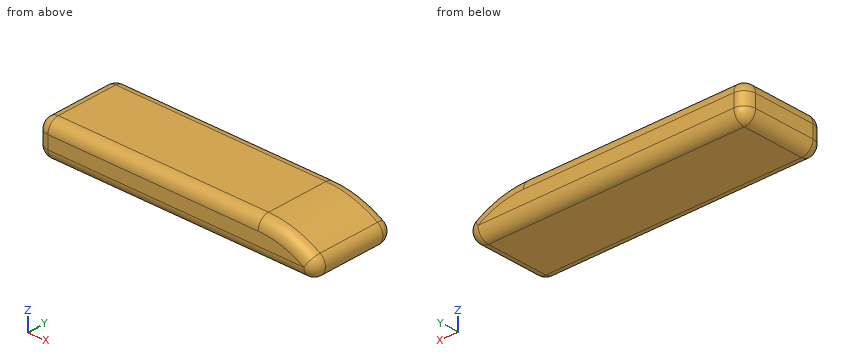
```python
from build123d import *

# Parameters (mm, degrees)
F1_DEPTH     = 38.1
F2_R         = 5.08
F3_F1_R      = 5.08
F3_T2_DEPTH  = 94.7599984092
F3_T4_DEPTH  = 115.3407412507
F3_S8_W      = 5.1816
F3_S8_H      = 5.1816
F3_T9_DEPTH  = 5.1816
F3_S14_W     = 5.1816
F3_S14_H     = 5.1816
F3_T15_DEPTH = 5.1816
F3_T19_ANGLE = 31.4774656297
F3_T21_ANGLE = 148.5225343703
F3_T22_DEPTH = 94.7599984092
F3_T24_DEPTH = 115.3407412507
F3_S28_W     = 5.1816
F3_S28_H     = 5.1816
F3_T29_DEPTH = 5.1816
F3_S34_W     = 5.1816
F3_S34_H     = 5.1816
F3_T35_DEPTH = 5.1816
F3_T39_ANGLE = 31.4774656297
F3_T41_ANGLE = 148.5225343703


# Not quite as in the source:
# - a fillet or chamfer that OpenCascade refuses, or shapes differently, is made with other operations: its cross-section is extruded or revolved along the edge and cut away or added


with BuildPart() as f1:
    # F0 (on Front) → F1 (new body)
    with BuildSketch(Plane.XZ):
        with BuildLine():
            Line((9.9600013345, 7.7700004913), (-89.8799970746, 7.7700004913))
            Line((-89.8799970746, 7.7700004913), (-89.8799970746, -8.1900004297))
            Line((-89.8799970746, -8.1900004297), (44.0999977291, -8.1900004297))
            ThreePointArc((44.0999977291, -8.1900004297), (28.8031763803, 3.5829980082), (9.9600013345, 7.7700004913))
        make_face()
    extrude(amount=F1_DEPTH)

    # F2
    f2_edges = [f1.edges().sort_by_distance(p)[0] for p in [
        (-89.879997, -19.05, -8.19),
        (-89.879997, 0, -0.21),
        (-89.879997, -19.05, 7.77),
        (-89.879997, -38.1, -0.21),
    ]]
    fillet(f2_edges, radius=F2_R)

    # F3: fillet of radius 5.08 on 12 edges, made by hand

    # F3_f1
    f3_f1_edges = [f1.edges().sort_by_distance(p)[0] for p in [
        (44.0999977291, -19.05, -8.1900004297),
    ]]
    fillet(f3_f1_edges, radius=F3_F1_R)

    # F3_s3 → F3_t2 (cut)
    with BuildSketch(Plane.YZ.offset(-84.7999970746)):
        with BuildLine():
            ThreePointArc((0, 2.6900004913), (-1.4878975516, 6.2821029397), (-5.08, 7.7700004913))
            Line((-5.08, 7.7700004913), (-5.08, 7.8716004913))
            Line((-5.08, 7.8716004913), (0.1016, 7.8716004913))
            Line((0.1016, 7.8716004913), (0.1016, 2.6900004913))
            Line((0.1016, 2.6900004913), (0, 2.6900004913))
        make_face()
    extrude(amount=F3_T2_DEPTH, mode=Mode.SUBTRACT)

    # F3_s5 → F3_t4 (cut)
    with BuildSketch(Plane.YZ.offset(-84.7999970746)):
        with BuildLine():
            ThreePointArc((0, -3.1100004297), (-1.4878975516, -6.7021028782), (-5.08, -8.1900004297))
            Line((-5.08, -8.1900004297), (-5.08, -8.2916004297))
            Line((-5.08, -8.2916004297), (0.1016, -8.2916004297))
            Line((0.1016, -8.2916004297), (0.1016, -3.1100004297))
            Line((0.1016, -3.1100004297), (0, -3.1100004297))
        make_face()
    extrude(amount=F3_T4_DEPTH, mode=Mode.SUBTRACT)


with BuildPart() as f3_tool7:
    # F3_s8 → F3_t9 (new body)
    with BuildSketch(Plane.XZ.offset(5.08)):
        with Locations((-87.3907970746, 5.2808004913)):
            Rectangle(F3_S8_W, F3_S8_H)
    extrude(amount=-F3_T9_DEPTH)

    # F3_s10 → F3_t11 (revolve, cut)
    with BuildSketch(Plane(origin=(-84.7999970746, -5.08, 2.6900004913), x_dir=(0.7071067812, 0, -0.7071067812), z_dir=(0.7071067812, 0, 0.7071067812))):
        with BuildLine():
            ThreePointArc((0, -5.08), (5.08, 0), (0, 5.08))
            Line((0, 5.08), (0, -5.08))
        make_face()
    revolve(axis=Axis((-84.7999970746, -5.08, 2.6900004913), (0, 1, 0)), mode=Mode.SUBTRACT)


with BuildPart() as f1_1:
    add(f1.part)

    # F3_t6: cut F3_tool7
    add(f3_tool7.part, mode=Mode.SUBTRACT)


with BuildPart() as f3_tool13:
    # F3_s14 → F3_t15 (new body)
    with BuildSketch(Plane.XZ.offset(5.08)):
        with Locations((-87.3907970746, -5.7008004297)):
            Rectangle(F3_S14_W, F3_S14_H)
    extrude(amount=-F3_T15_DEPTH)

    # F3_s16 → F3_t17 (revolve, cut)
    with BuildSketch(Plane(origin=(-84.7999970746, -5.08, -3.1100004297), x_dir=(0.7071067812, 0, 0.7071067812), z_dir=(-0.7071067812, 0, 0.7071067812))):
        with BuildLine():
            ThreePointArc((0, -5.08), (5.08, 0), (0, 5.08))
            Line((0, 5.08), (0, -5.08))
        make_face()
    revolve(axis=Axis((-84.7999970746, -5.08, -3.1100004297), (0, 1, 0)), mode=Mode.SUBTRACT)


with BuildPart() as f1_2:
    add(f1_1.part)

    # F3_t12: cut F3_tool13
    add(f3_tool13.part, mode=Mode.SUBTRACT)

    # F3_s18 → F3_t19 (revolve, cut)
    with BuildSketch(Plane(origin=(23.5986358548, 0, -14.4484990421), x_dir=(0, 1, 0), z_dir=(0.8528455965, 0, -0.5221631818))):
        with BuildLine():
            ThreePointArc((0, 13.2949019826), (-1.4878975516, 16.887004431), (-5.08, 18.3749019826))
            Line((-5.08, 18.3749019826), (-5.08, 18.4765019826))
            Line((-5.08, 18.4765019826), (0.1016, 18.4765019826))
            Line((0.1016, 18.4765019826), (0.1016, 13.2949019826))
            Line((0.1016, 13.2949019826), (0, 13.2949019826))
        make_face()
    revolve(axis=Axis((9.9600013345, 0, -36.7243886458), (0, -1, 0)), revolution_arc=F3_T19_ANGLE, mode=Mode.SUBTRACT)

    # F3_s20 → F3_t21 (revolve, cut)
    with BuildSketch(Plane(origin=(23.5986358548, 0, -14.4484990421), x_dir=(0, 1, 0), z_dir=(-0.8528455965, 0, 0.5221631818))):
        with BuildLine():
            ThreePointArc((0, -13.2949019826), (-1.4878975516, -16.887004431), (-5.08, -18.3749019826))
            Line((-5.08, -18.3749019826), (-5.08, -18.4765019826))
            Line((-5.08, -18.4765019826), (0.1016, -18.4765019826))
            Line((0.1016, -18.4765019826), (0.1016, -13.2949019826))
            Line((0.1016, -13.2949019826), (0, -13.2949019826))
        make_face()
    revolve(axis=Axis((30.5407441761, 0, -3.1100004297), (0, 1, 0)), revolution_arc=F3_T21_ANGLE, mode=Mode.SUBTRACT)

    # F3_s23 → F3_t22 (cut)
    with BuildSketch(Plane.YZ.offset(-84.7999970746)):
        with BuildLine():
            ThreePointArc((-33.02, 7.7700004913), (-36.6121024484, 6.2821029397), (-38.1, 2.6900004913))
            Line((-38.1, 2.6900004913), (-38.2016, 2.6900004913))
            Line((-38.2016, 2.6900004913), (-38.2016, 7.8716004913))
            Line((-38.2016, 7.8716004913), (-33.02, 7.8716004913))
            Line((-33.02, 7.8716004913), (-33.02, 7.7700004913))
        make_face()
    extrude(amount=F3_T22_DEPTH, mode=Mode.SUBTRACT)

    # F3_s25 → F3_t24 (cut)
    with BuildSketch(Plane.YZ.offset(-84.7999970746)):
        with BuildLine():
            ThreePointArc((-33.02, -8.1900004297), (-36.6121024484, -6.7021028782), (-38.1, -3.1100004297))
            Line((-38.1, -3.1100004297), (-38.2016, -3.1100004297))
            Line((-38.2016, -3.1100004297), (-38.2016, -8.2916004297))
            Line((-38.2016, -8.2916004297), (-33.02, -8.2916004297))
            Line((-33.02, -8.2916004297), (-33.02, -8.1900004297))
        make_face()
    extrude(amount=F3_T24_DEPTH, mode=Mode.SUBTRACT)


with BuildPart() as f3_tool27:
    # F3_s28 → F3_t29 (new body)
    with BuildSketch(Plane.XY.offset(2.6900004913)):
        with Locations((-87.3907970746, -35.6108)):
            Rectangle(F3_S28_W, F3_S28_H)
    extrude(amount=F3_T29_DEPTH)

    # F3_s30 → F3_t31 (revolve, cut)
    with BuildSketch(Plane(origin=(-84.7999970746, -33.02, 2.6900004913), x_dir=(0.7071067812, 0.7071067812, 0), z_dir=(0.7071067812, -0.7071067812, 0))):
        with BuildLine():
            ThreePointArc((0, -5.08), (5.08, 0), (0, 5.08))
            Line((0, 5.08), (0, -5.08))
        make_face()
    revolve(axis=Axis((-84.7999970746, -33.02, 2.6900004913), (0, 0, 1)), mode=Mode.SUBTRACT)


with BuildPart() as f1_3:
    add(f1_2.part)

    # F3_t26: cut F3_tool27
    add(f3_tool27.part, mode=Mode.SUBTRACT)


with BuildPart() as f3_tool33:
    # F3_s34 → F3_t35 (new body)
    with BuildSketch(Plane.XY.offset(-3.1100004297)):
        with Locations((-87.3907970746, -35.6108)):
            Rectangle(F3_S34_W, F3_S34_H)
    extrude(amount=-F3_T35_DEPTH)

    # F3_s36 → F3_t37 (revolve, cut)
    with BuildSketch(Plane(origin=(-84.7999970746, -33.02, -3.1100004297), x_dir=(0.7071067812, 0.7071067812, 0), z_dir=(-0.7071067812, 0.7071067812, 0))):
        with BuildLine():
            ThreePointArc((0, -5.08), (5.08, 0), (0, 5.08))
            Line((0, 5.08), (0, -5.08))
        make_face()
    revolve(axis=Axis((-84.7999970746, -33.02, -3.1100004297), (0, 0, -1)), mode=Mode.SUBTRACT)


with BuildPart() as f1_4:
    add(f1_3.part)

    # F3_t32: cut F3_tool33
    add(f3_tool33.part, mode=Mode.SUBTRACT)

    # F3_s38 → F3_t39 (revolve, cut)
    with BuildSketch(Plane(origin=(23.5986358548, 0, -14.4484990421), x_dir=(0, 1, 0), z_dir=(0.8528455965, 0, -0.5221631818))):
        with BuildLine():
            ThreePointArc((-33.02, 18.3749019826), (-36.6121024484, 16.887004431), (-38.1, 13.2949019826))
            Line((-38.1, 13.2949019826), (-38.2016, 13.2949019826))
            Line((-38.2016, 13.2949019826), (-38.2016, 18.4765019826))
            Line((-38.2016, 18.4765019826), (-33.02, 18.4765019826))
            Line((-33.02, 18.4765019826), (-33.02, 18.3749019826))
        make_face()
    revolve(axis=Axis((9.9600013345, -38.1, -36.7243886458), (0, -1, 0)), revolution_arc=F3_T39_ANGLE, mode=Mode.SUBTRACT)

    # F3_s40 → F3_t41 (revolve, cut)
    with BuildSketch(Plane(origin=(23.5986358548, 0, -14.4484990421), x_dir=(0, 1, 0), z_dir=(-0.8528455965, 0, 0.5221631818))):
        with BuildLine():
            ThreePointArc((-33.02, -18.3749019826), (-36.6121024484, -16.887004431), (-38.1, -13.2949019826))
            Line((-38.1, -13.2949019826), (-38.2016, -13.2949019826))
            Line((-38.2016, -13.2949019826), (-38.2016, -18.4765019826))
            Line((-38.2016, -18.4765019826), (-33.02, -18.4765019826))
            Line((-33.02, -18.4765019826), (-33.02, -18.3749019826))
        make_face()
    revolve(axis=Axis((30.5407441761, -38.1, -3.1100004297), (0, 1, 0)), revolution_arc=F3_T41_ANGLE, mode=Mode.SUBTRACT)


solid = f1_4.part
```
Work out the finished part from the listing and answer in its coordinate system (mm). Round coordinates to 2 decimals unless told otherwise and drop trailing zeros. Loops run counter-clockwise (first coordinate to the right, second up) from the corner with the lowest first, then second, coordinate; pieces in that order, holes last.
(1) The part is cut by section A-A, the plane x = -9.5. Give the vertices of the cut face in (y, z), and give its area (3 significant figures).
Computed values:
outline: (-38.1, -3.11) arc R5.08 ccw to (-33.02, -8.19) - (-5.08, -8.19) arc R5.08 ccw to (0, -3.11) - (0, 2.69) arc R5.08 ccw to (-5.08, 7.77) - (-33.02, 7.77) arc R5.08 ccw to (-38.1, 2.69) - close
area: 586 mm2
(2) Each of these flat-tipped pins is pushed along its axis until it touches: P1, Ø8, axis at y = -18.5, z = 4.5, coming from the +X side; P2, Ø8, axis at y = -23.5, z = 3, coming from the +X side; P3, Ø2, axis at x = 19.5, y = -9.5, coming from the +Z side. Where does it stop, or does it pass through?
Computed values:
P1: stops at x = 34.11
P2: stops at x = 35.16
P3: stops at z = 6.94
(3) The part is cut by section B-B, the plane y = -11. Give the vertices of the cut face in (x, z).
Computed values:
outline: (-89.88, -3.11) arc R5.08 ccw to (-84.8, -8.19) - (30.54, -8.19) arc R5.08 ccw to (33.19, 1.22) arc R44.49 ccw to (9.96, 7.77) - (-84.8, 7.77) arc R5.08 ccw to (-89.88, 2.69) - close
(4) Find the intervals of material crossed by L1, parallel to X at y = -36, z = -6.5; L2, parallel to Y at x = -42, z = 7.25; L3, parallel to X at y = -28, z = -0.75, in increasing order.
Computed values:
L1: x = -87.13 to 32.87
L2: y = -35.26 to -2.84
L3: x = -89.88 to 35.04
